```python
from build123d import *

# Parameters (mm, degrees)
SKETCH1_R           = 3.175
BOSS_EXTRUDE1_DEPTH = 6.35
BOSS_EXTRUDE2_START = -6.35
SKETCH2_R           = 4.7625
BOSS_EXTRUDE2_DEPTH = 6.35


with BuildPart() as part:
    # Sketch1 → Boss-Extrude1 (new body)
    with BuildSketch(Plane(origin=(0, 0, 0), x_dir=(0, 0, -1), z_dir=(1, 0, 0))):
        with BuildLine():
            Line((-8.980256121, 8.980256121), (8.980256121, 26.940768363))
            ThreePointArc((8.980256121, 26.940768363), (26.940768363, 26.940768363), (26.940768363, 8.980256121))
            ThreePointArc((26.940768363, 8.980256121), (18.331397871, -3.512535502), (14.733533544, -18.2518189))
            ThreePointArc((14.733533544, -18.2518189), (3.99537448, -50.125222998), (-21.49411099, -72.068515352))
            ThreePointArc((-21.49411099, -72.068515352), (-38.413515352, -66.042425736), (-32.387425736, -49.123021375))
            ThreePointArc((-32.387425736, -49.123021375), (-13.857306444, -30.125859248), (-12.166610815, -3.641919999))
            ThreePointArc((-12.166610815, -3.641919999), (-12.313704877, 3.108483907), (-8.980256121, 8.980256121))
        make_face()
        Circle(SKETCH1_R, mode=Mode.SUBTRACT)
        with Locations((17.960512242, 17.960512242)):
            Circle(SKETCH1_R, mode=Mode.SUBTRACT)
        with Locations((-26.940768363, -60.595768363)):
            Circle(SKETCH1_R, mode=Mode.SUBTRACT)
    extrude(amount=BOSS_EXTRUDE1_DEPTH)

    # Sketch2 → Boss-Extrude2 (add)
    with BuildSketch(Plane(origin=(6.35, 0, 0), x_dir=(0, 0, -1), z_dir=(1, 0, 0)).offset(BOSS_EXTRUDE2_START)):
        with BuildLine():
            Line((-8.980256121, 8.980256121), (8.980256121, 26.940768363))
            ThreePointArc((8.980256121, 26.940768363), (19.47129419, 30.570331349), (28.80800074, 24.565207034))
            ThreePointArc((28.80800074, 24.565207034), (-11.744974479, 72.511118598), (-65.000542096, 105.785714805))
            ThreePointArc((-65.000542096, 105.785714805), (-109.616580791, 82.065642196), (-76.995649237, 43.476685512))
            ThreePointArc((-76.995649237, 43.476685512), (-36.623825936, 30.865592429), (-12.166610815, -3.641919999))
            ThreePointArc((-12.166610815, -3.641919999), (-12.313704877, 3.108483907), (-8.980256121, 8.980256121))
        make_face()
        with Locations((-77.740768363, 75.929231637)):
            Circle(SKETCH2_R, mode=Mode.SUBTRACT)
    extrude(amount=BOSS_EXTRUDE2_DEPTH)


solid = part.part
```
Design review of the part built by this model. Coordinates are the model's own, in mm. Round coordinates to 2 decimals unless told otherwise and drop trailing zeros. Write each loop counter-clockwise with the first axis right and the second up, starting at its lowest first coordinate (ties: lowest second). Pieces come first, ordered by that corner, then holes.
Item 1: Clearance check with flat-ended pins moving along their axes: pin 1 Ø1 at (x, y) = (3.5, -40) entering from +Z; pin 2 Ø10 at (y, z) = (-60.6, 26.94) entering from +X; pin 3 Ø2 at (x, y) = (4.5, -17.5) entering from -Z; pin 4 Ø1 at (x, z) = (5.5, 35) entering from +Y. State where each tip first meets the part, or that it passes through.
Item 2: For probe 1 along Y at (x, z) = (5, 29.5); probe 2 along Z at (x, y) = (5.5, -62.5); probe 3 along Z at (x, y) = (2.5, -1), list the stretches that pass through material, from the lowest coordinate up.
Item 3: We need section A-A on z = 0. Write out the cut boundary in (x, y) (3 decimals).
Item 4: We need section C-C on z = 27.5. Write out the cut boundary in (x, y).
Item 5: We need section B-B on y = 0. Write out the cut boundary in (x, z) (3 decimals).
Item 6: We need section D-D on x = 5. State how many separate pieces and enclosed holes the cut face has, and give its area (3 significant figures).
Item 7: The part is to be moulded in two halves that separate along Z. For faces 1 (the cylindrical face through (3.13, -3.32, -18.42)), 2 (the flat face through (6.35, 39, 41)), 3 (the cylindrical face through (3.1, -63.7, 27.6)), say which applies: +Z half, -Z half, draft (parallel to the pull), parting line (faces both ways), or undercut.
Returned:
1. pin 1: stops at z = 20.68
1. pin 2: stops at x = 6.35
1. pin 3: stops at z = -14.87
1. pin 4: stops at y = 90.22
2. probe 1: y = -73.04 to -62.47, -58.72 to -47.6, 24.88 to 86.24
2. probe 2: z = 6.91 to 24.4, 29.48 to 39.5
2. probe 3: z = -19.56 to -3.01, 3.01 to 13.02
3. outline: (0, -55.438) - (6.35, -55.438) - (6.35, -3.175) - (0, -3.175) - close; (0, 3.175) - (6.35, 3.175) - (6.35, 61.498) - (0, 61.498) - close
4. outline: (0, -73.28) - (6.35, -73.28) - (6.35, -63.72) - (0, -63.72) - close; (0, -57.47) - (6.35, -57.47) - (6.35, -46.34) - (0, -46.34) - close; (0, 22.86) - (6.35, 22.86) - (6.35, 84.85) - (0, 84.85) - close
5. outline: (0, -20.109) - (6.35, -20.109) - (6.35, -3.175) - (0, -3.175) - close; (0, 3.175) - (6.35, 3.175) - (6.35, 13.373) - (0, 13.373) - close
6. separate pieces: 1
6. enclosed holes: 4
6. area: 9,810 mm2
7. face 1: -Z half
7. face 2: draft
7. face 3: undercut
